Autodesk Fusion 360 part; units mm, degrees
sketch "Sketch1" plane through (0, 0, 0) normal (0, 0, 1) x (1, 0, 0)
  circle A0 centre (0, 0) radius 28.5
  dimension "d1" = 57
extrude "Extrude1" add sketch "Sketch1" along normal blind 150
sketch "Sketch2" plane through (0, 0, 0) normal (0, 0, -1) x (1, 0, 0)
  circle A0 centre (0, 0) radius 28.5
  circle A1 centre (0, 0) radius 27
  dimension "d4" = 54
extrude "Extrude2" cut sketch "Sketch2" against normal blind 530 contours A1
sketch "Sketch3" plane through (0, 0, 0) normal (0, 1, 0) x (1, 0, 0)
  line L0 (0, 0) -> (20, 0)
  line L1 (20, 0) -> (20, -5)
  line L2 (20, -5) -> (-20, -5)
  line L3 (-20, -5) -> (-20, -10)
  line L4 (-20, -10) -> (20, -10)
  line L5 (20, -10) -> (20, -5)
  dimension "d7" = 20
  dimension "d8" = 40
  dimension "d9" = 5
  dimension "d10" = 5
extrude "Extrude3" cut sketch "Sketch3" along normal blind 50 and the other way blind 35
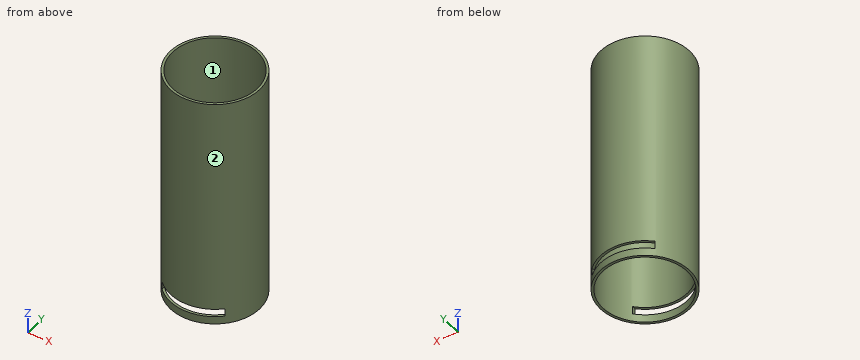
Geometry: final body of the model. Coordinates: model frame, mm. Face numbers are marked on the shaded views. Give positions to 0.01 mm unless a question says otherwise; leave off trailing zeros. Write each loop counter-clockwise with the first axis right and the second up, starting at its lowest first coordinate (ties: lowest second). Pieces come first, ordered by that corner, then holes. Notation, with made-up numbers: (-36, 84) -> (16, 84) arc R22 ccw to (16, 107) -> close; hole circle Ø7 at (-19, 56.25). An arc over 180 degrees is marked (long way). Answer as a JSON object with one key per item and string values.
1. Cut plane C-C on x = -24.5. Output: boundary loops of the cut face in (y, z).
Ans:
{"outline": "(-14.56, 0) -> (-11.35, 0) -> (-11.35, 150) -> (-14.56, 150) -> close; (11.35, 0) -> (14.56, 0) -> (14.56, 150) -> (11.35, 150) -> close"}
2. Mould query, pull axis X, two halves, no side actions, for the marked faces 1 and 2. Classes: pulls with the +X half, pulls with the -X half, needs draft (parallel to the pull), parting line crosses it, or undercut.
Ans:
{"face 1": "undercut", "face 2": "parting line crosses it"}
3. Cut plane B-B on y = 0. Output: boundary loops of the cut face in (x, z), and give its area (3 significant figures).
Ans:
{"outline": "(-28.5, 0) -> (-27, 0) -> (-27, 150) -> (-28.5, 150) -> close; (27, 0) -> (28.5, 0) -> (28.5, 150) -> (27, 150) -> close", "area": "450 mm^2"}
4. Ray query, probe 1 along Y at (x, z) = (0, 36); probe 2 along Y at (x, z) = (10, 98). Return the intervals inside material, ascending. Write a range as from..to.
Ans:
{"probe 1": "y = -28.5..-27, 27..28.5", "probe 2": "y = -26.69..-25.08, 25.08..26.69"}
5. Cut plane D-D on y = -24. Output: boundary loops of the cut face in (x, z), and give its area (3 significant figures).
Ans:
{"outline": "(-15.37, 0) -> (-12.37, 0) -> (-12.37, 5) -> (-15.37, 5) -> close; (-15.37, 10) -> (-12.37, 10) -> (-12.37, 150) -> (-15.37, 150) -> close; (12.37, 0) -> (15.37, 0) -> (15.37, 5) -> (12.37, 5) -> close; (12.37, 10) -> (15.37, 10) -> (15.37, 150) -> (12.37, 150) -> close", "area": "870 mm^2"}
6. Contact query for flat-ended pins moving along their axis: pin 1 (1 mm diameter, centred on y = 21, z = 127, fed in from -X); pin 2 (1.1 mm diameter, centred on y = -19, z = 6.5, fed in from +X); pin 3 (2.5 mm diameter, centred on y = 19, z = 7, fed in from +X). Output: stop coordinate, or through.
Ans:
{"pin 1": "stops at x = -19.8", "pin 2": "stops at x = 21.72", "pin 3": "stops at x = 22.3"}
7. Cut plane A-A on x = 0. Output: boundary loops of the cut face in (y, z).
Ans:
{"outline": "(-28.5, 0) -> (-27, 0) -> (-27, 5) -> (-28.5, 5) -> close; (-28.5, 10) -> (-27, 10) -> (-27, 150) -> (-28.5, 150) -> close; (27, 0) -> (28.5, 0) -> (28.5, 5) -> (27, 5) -> close; (27, 10) -> (28.5, 10) -> (28.5, 150) -> (27, 150) -> close"}
